from build123d import *

# Parameters (mm, degrees)
BOSS_EXTRU_1_DEPTH      = 1.5
BOSS_EXTRU_2_DEPTH      = 13.5
D_GAGEMENT_M32_D        = 3.4
D_GAGEMENT_M32_DEPTH    = 10
D_GAGEMENT_M32_TIP      = 1.021463052
D_GAGEMENT_M31_D        = 3.4
D_GAGEMENT_M31_DEPTH    = 10
D_GAGEMENT_M31_TIP      = 1.021463052
ESQUISSE12_W            = 13.5
ESQUISSE12_H            = 13.5
ENL_V_MAT_EXTRU_1_DEPTH = 1.5
CONG_1_R                = 1
CONG_2_R                = 1


# Some blends are built 0.0001 mm under size
with BuildPart() as part:
    # Esquisse2 → Boss.-Extru.1 (new body)
    with BuildSketch(Plane.XY.offset(1.5)):
        Polygon((-25.392437762, 124.305889048), (-178.410591433, 124.305889048), (-178.410591433, 149.305889048), (-222.374284091, 149.305889048), (-222.374284091, 124.305889048), (-375.392437762, 124.305889048), (-375.392437762, 109.305889048), (-207.374284091, 109.305889048), (-207.374284091, 134.305889048), (-193.410591433, 134.305889048), (-193.410591433, 109.305889048), (-25.392437762, 109.305889048), align=None)
    extrude(amount=BOSS_EXTRU_1_DEPTH)

    # Esquisse3 → Boss.-Extru.2 (add)
    with BuildSketch(Plane.XY.offset(3)):
        Polygon((-375.392437762, 122.805889048), (-220.874284091, 122.805889048), (-220.874284091, 147.805889048), (-179.910591433, 147.805889048), (-179.910591433, 122.805889048), (-25.392437762, 122.805889048), (-25.392437762, 124.305889048), (-178.410591433, 124.305889048), (-178.410591433, 149.305889048), (-222.374284091, 149.305889048), (-222.374284091, 124.305889048), (-375.392437762, 124.305889048), align=None)
    extrude(amount=BOSS_EXTRU_2_DEPTH)

    # Dégagement M32
    with Locations(Plane(origin=(-229.874284091, 116.805889048, 3), x_dir=(1, 0, 0), z_dir=(0, 0, 1))):
        with Locations((0, 0), (-70.518153671, 0), (-138.018153671, 0), (58.963692658, 0), (129.481846329, 0), (196.981846329, 0)):
            Hole(D_GAGEMENT_M32_D / 2, depth=D_GAGEMENT_M32_DEPTH)
            with Locations((0, 0, -(D_GAGEMENT_M32_DEPTH + D_GAGEMENT_M32_TIP / 2))):  # 118° drill point
                Cone(0, D_GAGEMENT_M32_D / 2, D_GAGEMENT_M32_TIP, mode=Mode.SUBTRACT)

    # Dégagement M31
    with Locations(Plane(origin=(-214.874284091, 137.305889048, 3), x_dir=(1, 0, 0), z_dir=(0, 0, 1))):
        with Locations((0, 0), (28.963692658, 0)):
            Hole(D_GAGEMENT_M31_D / 2, depth=D_GAGEMENT_M31_DEPTH)
            with Locations((0, 0, -(D_GAGEMENT_M31_DEPTH + D_GAGEMENT_M31_TIP / 2))):  # 118° drill point
                Cone(0, D_GAGEMENT_M31_D / 2, D_GAGEMENT_M31_TIP, mode=Mode.SUBTRACT)

    # Esquisse12 → Enlèv. mat.-Extru.1 (cut)
    with BuildSketch(Plane.XY.offset(3)):
        with Locations((-214.124284091, 116.055889048)):
            Rectangle(ESQUISSE12_W, ESQUISSE12_H)
        with Locations((-186.660591433, 116.055889048)):
            Rectangle(ESQUISSE12_W, ESQUISSE12_H)
    extrude(amount=-ENL_V_MAT_EXTRU_1_DEPTH, mode=Mode.SUBTRACT)

    # Congé1
    # the kernel refuses this fillet: 1 mm, written as the material it adds along each edge
    with BuildSketch(Plane(origin=(-179.910591433, 122.805889048, 3), x_dir=(0, -1, 0), z_dir=(1, 0, 0))) as cong_1_piece_1:
        with BuildLine():
            CenterArc((CONG_1_R, -CONG_1_R), CONG_1_R, 90, 90)
            Line((0, -CONG_1_R), (0, 0))
            Line((0, 0), (CONG_1_R, 0))
        make_face()
    extrude(amount=154.518153671)
    with BuildSketch(Plane(origin=(-223.374284091, 147.805889048, 3), x_dir=(0, 0, 1), z_dir=(1, 0, 0))) as cong_1_piece_2_section:
        with BuildLine():
            CenterArc((CONG_1_R, CONG_1_R), CONG_1_R, 180, 90)
            Line((0, CONG_1_R), (0, 0))
            Line((0, 0), (CONG_1_R, 0))
        make_face()
    cong_1_piece_2 = extrude(amount=43.463692658, mode=Mode.PRIVATE)
    cong_1_piece_2 = split(cong_1_piece_2, bisect_by=Plane(origin=(-222.374284091, 147.582521109, 3.223367939), z_dir=(1, 0, 0)), keep=Keep.TOP, mode=Mode.PRIVATE)
    add(cong_1_piece_2)
    with BuildSketch(Plane(origin=(-375.392437762, 122.805889048, 3), x_dir=(0, 0, 1), z_dir=(1, 0, 0))) as cong_1_piece_3:
        with BuildLine():
            CenterArc((CONG_1_R, CONG_1_R), CONG_1_R, 180, 90)
            Line((0, CONG_1_R), (0, 0))
            Line((0, 0), (CONG_1_R, 0))
        make_face()
    extrude(amount=154.518153671)

    # Congé2
    cong_2_edges = [part.edges().sort_by_distance(p)[0] for p in [
        (-179.910591433, 134.805889048, 3),
        (-179.910591433, 147.512995829, 3.292893219),
        (-220.874284091, 147.512995829, 3.292893219),
        (-220.874284091, 134.805889048, 3),
        (-220.874284091, 147.805889048, 10.25),
        (-179.910591433, 147.805889048, 10.25),
    ]]
    fillet(cong_2_edges, radius=CONG_2_R - 0.0001)  # a hair under: the kernel refuses the full size


solid = part.part
Input: part model. Units: mm. Frame: model coordinates. A direction names the side the tool comes from. Coordinates: 2 decimals unless noted, no trailing zeros. Loops run counter-clockwise (first coordinate to the right, second up) from the corner with the lowest first, then second, coordinate; pieces in that order, holes last.
(1) First-contact query: pin 1 Ø5 at (x, z) = (-188, 9.5) entering from -Y; pin 2 Ø4 at (y, z) = (127.5, 14) entering from -X; pin 3 Ø4 at (x, y) = (-185.91, 137.31) entering from +Z. Flat tips, straight axial feed; report the tip coordinate or a pass-through.
(2) Set-up query: faces 4 (the face through (-222.374, 137, 9)), 5 (the face through (-201, 135, 3)), 6 (the face through (-104, 116, 3)), 7 (the face through (-200, 149.306, 9)), 8 (the face through (-178.411, 137, 9)). Return all of +Z, -Z, +X, -X, +Y, -Y with unobstructed straight access to the full face (end or side cutting, diameter ignored); none if empty.
(3) Section B-B on z = 7.5. Return the cut outline in (x, y), then the cut area to 3 significant figures.
(4) Pull-direction query (X, two-part tool) for faces 1 (the face through (-104, 122.806, 10)), 2 (the face through (-220.874, 132, 9)), 3 (the face through (-25.392, 119.55, 2.85)); classes: released by +X, released by -X, zero draft, split by the parting line, or undercut.
(5) Material intervals for probe 1 along X at (y, z) = (123.5, 6); probe 2 along X at (y, z) = (141.5, 9.25); probe 3 along Y at (x, z) = (-101, 14.75), sorted ascending.
(6) Section A-A on x = -80. Return the cut outline in (y, z).
Data:
1. pin 1: stops at y = 147.81
1. pin 2: stops at x = -222.37
1. pin 3: stops at z = 3
2. face 4: +Z, -Z, -X, +Y
2. face 5: +Z, -Y
2. face 6: +Z, +X, -X, -Y
2. face 7: +Z, -Z, +X, -X, +Y
2. face 8: +Z, -Z, +X, +Y
3. outline: (-375.39, 122.81) - (-220.87, 122.81) - (-220.87, 146.81) arc R1 cw to (-219.87, 147.81) - (-180.91, 147.81) arc R1 cw to (-179.91, 146.81) - (-179.91, 122.81) - (-25.39, 122.81) - (-25.39, 124.31) - (-178.41, 124.31) - (-178.41, 149.31) - (-222.37, 149.31) - (-222.37, 124.31) - (-375.39, 124.31) - close
3. area: 600 mm2
4. face 1: zero draft
4. face 2: undercut
4. face 3: released by +X
5. probe 1: x = -375.39 to -220.87, -179.91 to -25.39
5. probe 2: x = -222.37 to -220.87, -179.91 to -178.41
5. probe 3: y = 122.81 to 124.31
6. outline: (109.31, 1.5) - (124.31, 1.5) - (124.31, 16.5) - (122.81, 16.5) - (122.81, 4) arc R1 cw to (121.81, 3) - (109.31, 3) - close
